Check sheet for the modelled part. Datum: model origin and axes. Units: mm. Round coordinates to 2 decimals unless told otherwise and drop trailing zeros. Loops run counter-clockwise (first coordinate to the right, second up) from the corner with the lowest first, then second, coordinate; pieces in that order, holes last. Notation, with made-up numbers: (27.5, 15) - (52.5, 15) arc R31 cw to (52.5, 41) - close; hole circle Ø5 at (64.25, -22). An arc over 180 degrees is marked (long way). Answer in a Markdown table with one row per item. Add a question column.
(1) Thickness scan on line 1 along Y through (x, z) = (-77, -2.4); line 2 along X through (y, z) = (34.2, -1.8); line 3 along Y through (x, z) = (46, -1.3). Record the ranges inside material, lowest first.
(2) Cross-section at A-A on x = -26.5. Enter the section's corners in (y, z), then the cut area to 3 significant figures.
(3) Gauge pin test, flat end, axial feed: pin 1 (12 mm diameter, centred on x = 5.5, y = -94, fed in from -Z). Record the tip position at first contact, or that the pin passes through.
(4) Cross-section at B-B on x = 44. Enter the section's corners in (y, z).
(5) Cross-section at C-C on z = -2.85. Count the separate pieces of the cut face and the enclosed holes in it, then the cut area to 3 significant figures.
Autodesk Inventor part; units mm, degrees
ref_plane "YZ Plane" through (0, 0, 0) normal (1, 0, 0) x (0, 1, 0)
ref_plane "XZ Plane" through (0, 0, 0) normal (0, 1, 0) x (-1, 0, 0)
ref_plane "XY Plane" through (0, 0, 0) normal (0, 0, 1) x (1, 0, 0)
sketch "Sketch1" plane through (0, 0, 0) normal (0, 0, 1) x (1, 0, 0)
  line L0 (93.3916, -12.6) -> (93.3916, 12.6)
  line L1 (53.9763, -12.6) -> (93.3916, -12.6)
  line L2 (53.9763, -15.2) -> (53.9763, -12.6)
  line L3 (38.2753, -15.2) -> (53.9763, -15.2)
  line L4 (38.2753, -15.2) -> (23.4296, -15.2)
  line L5 (23.4296, -12.6) -> (23.4296, -15.2)
  line L6 (-76.0546, -12.6) -> (23.4296, -12.6)
  line L7 (23.4296, 12.6) -> (-76.0546, 12.6)
  line L8 (23.4296, 15.2) -> (23.4296, 12.6)
  line L9 (-76.0546, 12.6) -> (-76.0546, -12.6)
  line L10 (-70.1, 10) -> (-66.9, 10)
  line L11 (-66.9, -10) -> (-70.1, -10)
  line L12 (23.4296, 15.2) -> (53.9763, 15.2)
  line L13 (53.9763, 15.2) -> (53.9763, 12.6)
  line L14 (53.9763, 12.6) -> (93.3916, 12.6)
  line L15 (-77.0546, 13.6) -> (22.4296, 13.6)
  line L16 (22.4296, 13.6) -> (22.4296, 16.2)
  line L17 (22.4296, 16.2) -> (54.9763, 16.2)
  line L18 (54.9763, 16.2) -> (54.9763, 13.6)
  line L19 (54.9763, 13.6) -> (94.3916, 13.6)
  line L20 (94.3916, 13.6) -> (94.3916, -13.6)
  line L21 (94.3916, -13.6) -> (54.9763, -13.6)
  line L22 (54.9763, -13.6) -> (54.9763, -16.2)
  line L23 (54.9763, -16.2) -> (38.2753, -16.2)
  line L24 (38.2753, -16.2) -> (22.4296, -16.2)
  line L25 (22.4296, -16.2) -> (22.4296, -13.6)
  line L26 (22.4296, -13.6) -> (-77.0546, -13.6)
  line L27 (-77.0546, -13.6) -> (-77.0546, 13.6)
  line L28 (22.4296, -16.2) -> (22.4296, -20.2) construction
  line L29 (22.4296, -20.2) -> (-87.5704, -20.2)
  line L30 (-87.5704, -20.2) -> (-87.5704, 20.2)
  line L31 (-87.5704, 20.2) -> (22.4296, 20.2)
  line L32 (104.4296, -20.2) -> (22.4296, -20.2)
  line L33 (22.4296, 20.2) -> (104.4296, 20.2)
  line L34 (104.4296, 20.2) -> (104.4296, -20.2)
  dimension "d0" = 1
  dimension "d1" = 4
  dimension "d2" = 110
  dimension "d3" = 40.4
  dimension "d5" = 82
extrude "Extrusion1" add sketch "Sketch1" against normal blind 3.5 contours L29 L30 L31 L33 L34 L32
pattern_linear "Rectangular Pattern1" count 4 spacing 40.4 along (0, -1, 0)
sketch "Sketch2" plane through (-87.5704, 20.2, 0) normal (0, 1, 0) x (1, 0, 0)
  line L0 (192, 3.5) -> (192, 0)
  line L1 (192, 0) -> (0, 0)
  line L2 (0, 0) -> (0, 3.5)
  line L3 (0, 3.5) -> (192, 3.5)
  point P0 (87.5704, 0)
extrude "Extrusion2" add sketch "Sketch2" along normal blind 20
sketch "Sketch3" plane through (-87.5704, -141.4, 0) normal (0, -1, 0) x (1, 0, 0)
  line L0 (192, 0) -> (192, -3.5)
  line L1 (192, -3.5) -> (0, -3.5)
  line L2 (0, -3.5) -> (0, 0)
  line L3 (0, 0) -> (192, 0)
  point P0 (87.5704, 0)
extrude "Extrusion3" add sketch "Sketch3" along normal blind 20
sketch "Sketch4" plane through (0, 0, -3.5) normal (0, 0, -1) x (-1, 0, 0)
  line L0 (87.5704, -161.4) -> (-104.4296, -161.4)
  line L1 (87.5704, -161.4) -> (81.5704, -161.4)
  line L2 (81.5704, -161.4) -> (81.5704, 40.2)
  line L3 (-104.4296, 40.2) -> (87.5704, 40.2)
  line L4 (81.5704, -161.4) -> (81.5704, -155.4)
  line L5 (81.5704, 40.2) -> (81.5704, 34.2)
  line L6 (77.0546, -107.6) -> (-22.4296, -107.6)
  line L7 (77.0546, -67.2) -> (77.0546, -94.4)
  line L8 (77.0546, -107.6) -> (77.0546, -94.4)
  line L9 (77.0546, -101) -> (81.5704, -101)
  line L10 (77.0546, -67.2) -> (77.0546, -53.8327)
  line L11 (77.0546, -60.5163) -> (81.5704, -60.6)
  line L12 (77.0546, -54) -> (77.0546, -26.8)
  line L13 (77.0546, -26.8) -> (77.0546, -13.3059)
  line L14 (77.0546, -20.0529) -> (81.5704, -20.0529)
  line L15 (-94.3916, -107.6) -> (-54.9763, -107.6)
  line L16 (-94.3916, -67.2) -> (-94.3916, -94.4)
  line L17 (-94.3916, -107.6) -> (-94.3916, -94.4)
  line L18 (-54.9763, -54) -> (-94.3916, -54)
  line L19 (-94.3916, -67.2) -> (-94.3916, -54)
  line L20 (-54.9763, -13.6) -> (-94.3916, -13.6)
  line L21 (-94.3916, -13.6) -> (-94.3916, 13.6)
  line L22 (-94.3916, -13.6) -> (-94.3916, 13.6)
  line L23 (-104.4296, -161.4) -> (-98.4296, -161.4)
  line L24 (-98.4296, -161.4) -> (-98.4296, 40.2)
  line L25 (-94.3916, -101) -> (-98.4296, -101)
  line L26 (-94.3916, -60.6) -> (-98.4296, -60.6)
  line L27 (-94.3916, -26.8) -> (-94.3916, -13.6)
  line L28 (-94.3916, -20.2) -> (-98.4296, -20.2)
  line L29 (-98.4296, 40.2) -> (-98.4296, 34.2)
  line L30 (-98.4296, -161.4) -> (-98.4296, -155.4)
  point P0 (0, 0)
  dimension "d15" = 6
  dimension "d16" = 6
  dimension "d17" = 6
  dimension "d18" = 6
  dimension "d19" = 6
  dimension "d20" = 6
hole "Hole1" at (98.4296, -155.4, -3.5) at (98.4296, -155.4, -3.5) at (98.4296, -101, -3.5) at (98.4296, -60.6, -3.5) at (98.4296, -20.2, -3.5) at (98.4296, 34.2, -3.5) at (-81.5704, 34.2, -3.5) at (-81.5704, -20.0529, -3.5) at (-81.5704, -60.6, -3.5) at (-81.5704, -101, -3.5) at (-81.5704, -155.4, -3.5) direction (0, 0, 1) diameter 3.4 end through all
properties part number "UnderPlate-4x1"
Answers:
| question | item | result |
|---|---|---|
| 1 | line 1 | y = -161.4 to -134.8, -107.6 to -94.4, -67.2 to -54, -26.8 to -13.6, 13.6 to 40.2 |
| 1 | line 2 | x = -87.57 to -83.27, -79.87 to 96.73, 100.13 to 104.43 |
| 1 | line 3 | y = -161.4 to -137.4, -105 to -97, -64.6 to -56.6, -24.2 to -16.2, 16.2 to 40.2 |
| 2 | outline | (-161.4, -3.5) - (-134.8, -3.5) - (-134.8, 0) - (-161.4, 0) - close; (-107.6, -3.5) - (-94.4, -3.5) - (-94.4, 0) - (-107.6, 0) - close; (-67.2, -3.5) - (-54, -3.5) - (-54, 0) - (-67.2, 0) - close; (-26.8, -3.5) - (-13.6, -3.5) - (-13.6, 0) - (-26.8, 0) - close; (13.6, -3.5) - (40.2, -3.5) - (40.2, 0) - (13.6, 0) - close |
| 2 | area | 325 mm^2 |
| 3 | pin 1 | stops at z = -3.5 |
| 4 | outline | (-161.4, -3.5) - (-137.4, -3.5) - (-137.4, 0) - (-161.4, 0) - close; (-105, -3.5) - (-97, -3.5) - (-97, 0) - (-105, 0) - close; (-64.6, -3.5) - (-56.6, -3.5) - (-56.6, 0) - (-64.6, 0) - close; (-24.2, -3.5) - (-16.2, -3.5) - (-16.2, 0) - (-24.2, 0) - close; (16.2, -3.5) - (40.2, -3.5) - (40.2, 0) - (16.2, 0) - close |
| 5 | separate pieces | 1 |
| 5 | enclosed holes | 14 |
| 5 | area | 19,300 mm^2 |
